Design review of the part shown in the three views and the two pictorial views. Dimensions are in mm from the part's minimum x, y and z. Round coordinates to 2 decimals unless told otherwise and drop trailing zeros. Loops run counter-clockwise (first coordinate to the right, second up) from the corner with the lowest first, then second, coordinate; pieces in that order, holes last. Notation, with made-up numbers: (24.25, 25) -> (30.25, 25) arc R33 cw to (30.25, 64) -> close; hole circle Ø2 at (-21, 67.5). An arc over 180 degrees is marked (long way). Use a Markdown table: item, result. Add a question column.
1) Insertion check: pin 1 (0.6 mm diameter, centred on y = 22, z = 1, fed in from +X); pin 2 (12 mm diameter, centred on x = 28, y = 19.5, fed in from -Z). Each pin has a flat end and moves straight along its axis. Give the tip position at first contact, or say it passes through.
2) Consider section A-A on y = 17.65. Give the boundary of the cut face in (x, z), plus the area to 3 significant figures.
3) Consider section B-B on x = 17.65. Give the boundary of the cut face in (y, z), plus the area to 3 significant figures.
4) Wall thickness on probe 1 along Y at (x, z) = (17.65, 0.7); probe 2 along X at (y, z) = (17, 1.8); probe 3 along X at (y, z) = (18.5, 0.9): over which ranges is each line inside the solid? List them lowest first.
5) Consider section C-C on z = 0.75. Give the boundary of the cut face in (x, y).
6) Consider section D-D on x = 2.15. Give the boundary of the cut face in (y, z), plus the area to 3 significant figures.
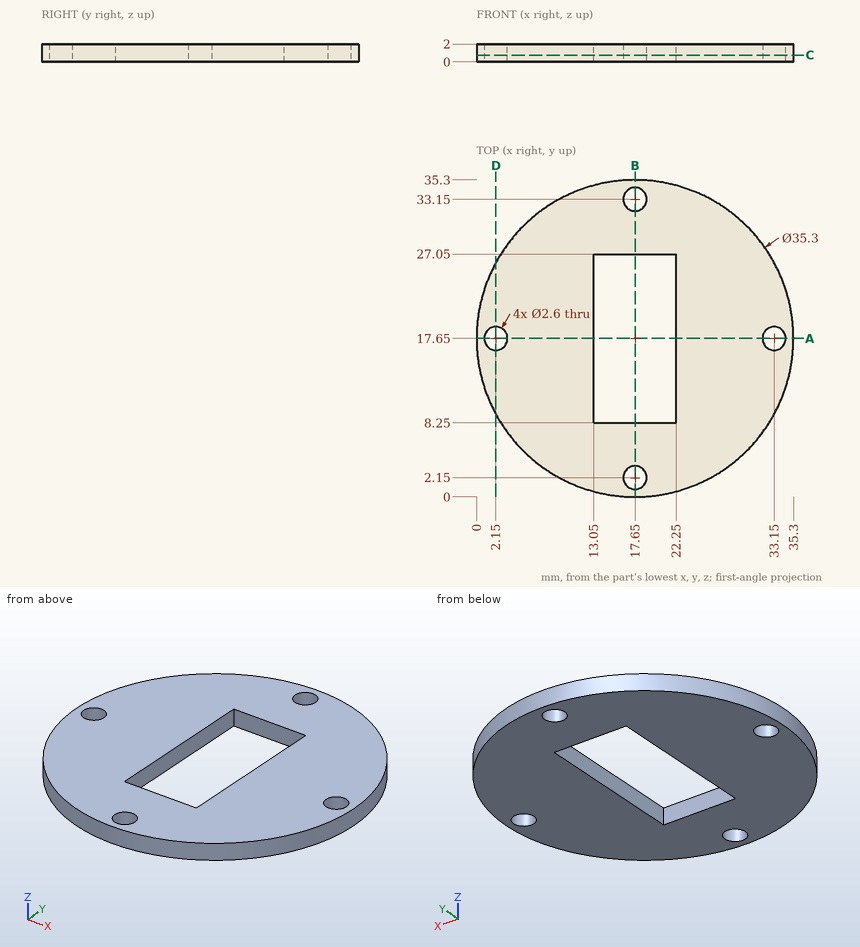
Result set:
| question | item | result |
|---|---|---|
| 1 | pin 1 | x = 34.83 |
| 1 | pin 2 | z = 0 |
| 2 | outline | (0, 0) -> (0.85, 0) -> (0.85, 2) -> (0, 2) -> close; (3.45, 0) -> (13.05, 0) -> (13.05, 2) -> (3.45, 2) -> close; (22.25, 0) -> (31.85, 0) -> (31.85, 2) -> (22.25, 2) -> close; (34.45, 0) -> (35.3, 0) -> (35.3, 2) -> (34.45, 2) -> close |
| 2 | area | 41.8 mm2 |
| 3 | outline | (0, 0) -> (0.85, 0) -> (0.85, 2) -> (0, 2) -> close; (3.45, 0) -> (8.25, 0) -> (8.25, 2) -> (3.45, 2) -> close; (27.05, 0) -> (31.85, 0) -> (31.85, 2) -> (27.05, 2) -> close; (34.45, 0) -> (35.3, 0) -> (35.3, 2) -> (34.45, 2) -> close |
| 3 | area | 22.6 mm2 |
| 4 | probe 1 | 0 to 0.85, 3.45 to 8.25, 27.05 to 31.85, 34.45 to 35.3 |
| 4 | probe 2 | 0.01 to 1.02, 3.28 to 13.05, 22.25 to 32.02, 34.28 to 35.29 |
| 4 | probe 3 | 0.02 to 1.17, 3.13 to 13.05, 22.25 to 32.17, 34.13 to 35.28 |
| 5 | outline | circle Ø35.3 at (17.65, 17.65); hole circle Ø2.6 at (2.15, 17.65); hole (13.05, 8.25) -> (22.25, 8.25) -> (22.25, 27.05) -> (13.05, 27.05) -> close; hole circle Ø2.6 at (17.65, 2.15); hole circle Ø2.6 at (17.65, 33.15); hole circle Ø2.6 at (33.15, 17.65) |
| 6 | outline | (9.21, 0) -> (16.35, 0) -> (16.35, 2) -> (9.21, 2) -> close; (18.95, 0) -> (26.09, 0) -> (26.09, 2) -> (18.95, 2) -> close |
| 6 | area | 28.6 mm2 |
